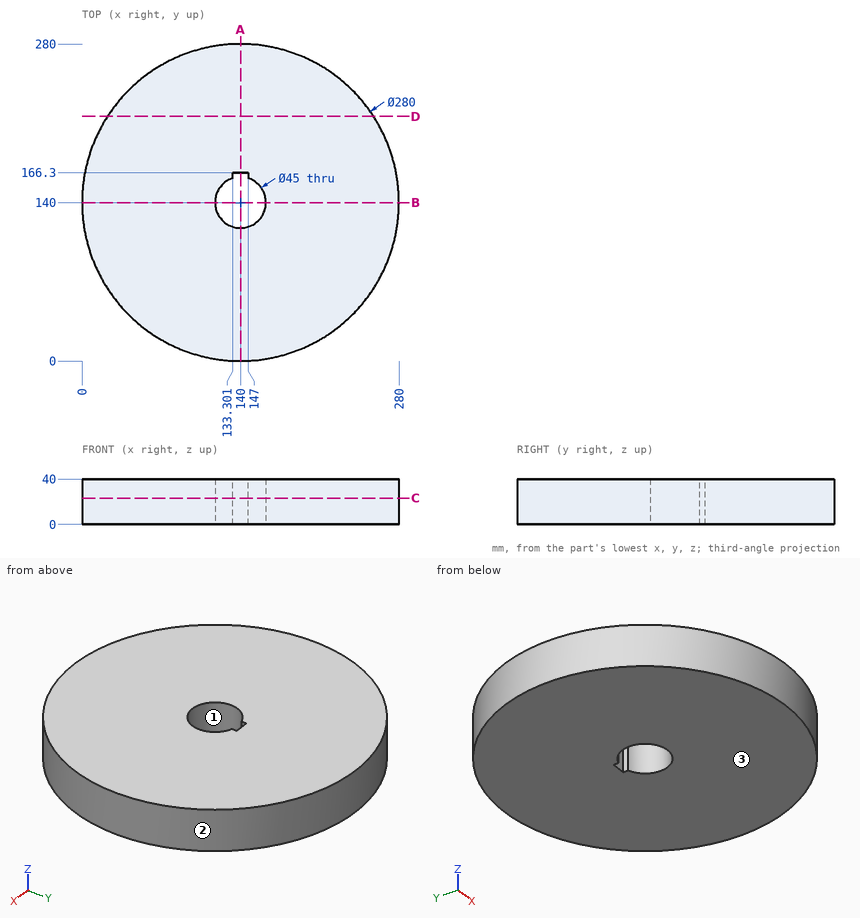
Geometry check sheet. Reference: drawing and pictorial views, mm from the part's lowest x, y, z. Coordinates: 2 decimals unless noted, no trailing zeros. Order: outer loops, then holes, each group sorted by start corner. A loop starts at its lowest first (then second) coordinate and runs counter-clockwise, first axis right, second up. Notation, with made-up numbers: (-37, 82.25) - (-7, 82.25) arc R17 ccw to (-7, 105.25) - close; hole circle Ø5 at (48, 58.25). An arc over 180 degrees is marked (long way). One line per item, written item: value.
(1) Sectioned sample at B-B (y = 140). Enter the section's corners in (x, z).
Data:
outline: (0, 0) - (117.5, 0) - (117.5, 40) - (0, 40) - close; (162.5, 0) - (280, 0) - (280, 40) - (162.5, 40) - close
(2) Thickness scan on probe 1 along Y at (x, z) = (137.5, 10); probe 2 along Y at (x, z) = (196.5, 10.5); probe 3 along Y at (x, z) = (63, 4). Record the ranges inside material, lowest first. Write a range as from..to.
Data:
probe 1: y = 0.02..117.64, 166.3..279.98
probe 2: y = 11.91..268.09
probe 3: y = 23.08..256.92
(3) Release check for a two-part mould opening along X. For the marked faces 1, 2 and 3 record: +X half, -X half, draft (parallel to the pull), parting line (faces both ways), or undercut.
Data:
face 1: undercut
face 2: parting line
face 3: draft
(4) Sectioned sample at D-D (y = 216). Enter the section's corners in (x, z) (1 decimal).
Data:
outline: (22.4, 0) - (257.6, 0) - (257.6, 40) - (22.4, 40) - close
(5) Depth check by flat-ended pin: pin 1 Ø1.5 at (x, z) = (199, 12) entering from -Y; pin 2 Ø12 at (y, z) = (171, 27.5) entering from +X; pin 3 Ø3 at (x, z) = (70, 33.5) entering from -Y. Enter the tip coordinate at first touch or a pass-through.
Data:
pin 1: stops at y = 12.69
pin 2: stops at x = 277.75
pin 3: stops at y = 17.9
(6) Sectioned sample at A-A (x = 140). Enter the section's corners in (y, z), and give its area (3 significant figures).
Data:
outline: (0, 0) - (117.5, 0) - (117.5, 40) - (0, 40) - close; (166.3, 0) - (280, 0) - (280, 40) - (166.3, 40) - close
area: 9,250 mm^2
(7) Sectioned sample at C-C (z = 23). Enter the section's corners in (x, y).
Data:
outline: circle Ø280 at (140, 140); hole (133.3, 161.48) arc R22.5 ccw (long way) to (147, 161.38) - (147, 166.3) - (133.3, 166.3) - close
